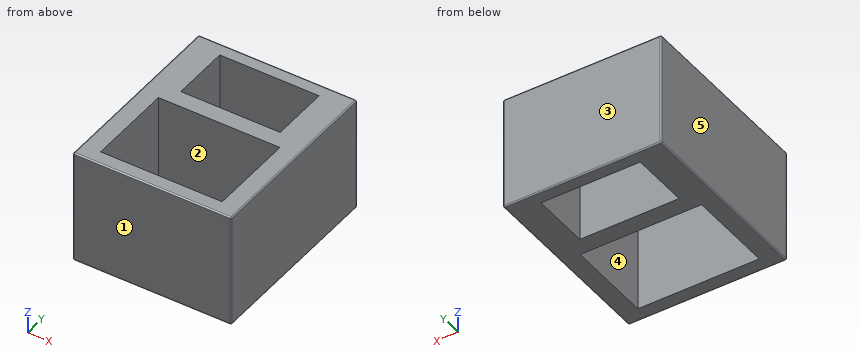
from build123d import *

# Parameters (mm, degrees)
SKETCH_1_W          = 250
SKETCH_1_H          = 300
EXTRUDE_1_DEPTH     = 180
FILLET_1_R          = 2
CUT_EXTRUDE_1_REACH = 432
SKETCH_2_W          = 157
SKETCH_2_H          = 93
SKETCH_2_W_2        = 192
SKETCH_2_H_2        = 138


with BuildPart() as part:
    # 草图1 → 凸台-拉伸1 (new body)
    with BuildSketch(Plane.XY):
        with Locations((125, 150)):
            Rectangle(SKETCH_1_W, SKETCH_1_H)
    extrude(amount=EXTRUDE_1_DEPTH)

    # 圆角1
    fillet_1_edges = [part.edges().sort_by_distance(p)[0] for p in [
        (250, 150, 180),
        (125, 300, 180),
        (0, 150, 180),
        (125, 300, 0),
        (250, 150, 0),
        (125, 0, 0),
        (0, 150, 0),
        (125, 0, 180),
        (0, 300, 90),
        (250, 300, 90),
        (250, 0, 90),
        (0, 0, 90),
    ]]
    fillet(fillet_1_edges, radius=FILLET_1_R)

    # 草图2 → 切除-拉伸1 (cut, up to next)
    with BuildSketch(Plane.XY.offset(180), mode=Mode.PRIVATE) as cut_extrude_1_sk1:
        with Locations((125, 233.5)):
            Rectangle(SKETCH_2_W, SKETCH_2_H)
    cut_extrude_1_tool1 = extrude(cut_extrude_1_sk1.sketch, amount=-CUT_EXTRUDE_1_REACH, mode=Mode.PRIVATE) & part.part
    # 草图2 → 切除-拉伸1 (cut, up to next)
    with BuildSketch(Plane.XY.offset(180), mode=Mode.PRIVATE) as cut_extrude_1_sk2:
        with Locations((125, 91)):
            Rectangle(SKETCH_2_W_2, SKETCH_2_H_2)
    cut_extrude_1_tool2 = extrude(cut_extrude_1_sk2.sketch, amount=-CUT_EXTRUDE_1_REACH, mode=Mode.PRIVATE) & part.part
    add(cut_extrude_1_tool1.solids().sort_by_distance((125, 233.5, 180))[0], mode=Mode.SUBTRACT)
    add(cut_extrude_1_tool2.solids().sort_by_distance((125, 91, 180))[0], mode=Mode.SUBTRACT)


solid = part.part
Model file for the job. Use its own axes, mm. Face numbers are marked on the shaded views. A direction names the side the tool comes from. Round coordinates to 2 decimals unless told otherwise and drop trailing zeros. Order: outer loops, then holes, each group sorted by start corner. A loop starts at its lowest first (then second) coordinate and runs counter-clockwise, first axis right, second up.
(1) Band-saw the part on C-C (z = 114). List the corners of the cut face in (x, y), then the cut area to 3 significant figures.
(2) Band-saw the part on D-D (x = 42.5). List the corners of the cut face in (y, z).
(3) Band-saw the part on A-A (y = 99). List the corners of the cut face in (x, z), then the cut area to 3 significant figures.
(4) 3-axis set-ups, long thin cutter, end or side, ignore diameter. For the marked faces 1 and 2: which of +Z, -Z, +X, -X, +Y, -Y reach the whole face in a straight line?
(5) Pull direction Y, two halves, no side cores. Call the marked faces 3, 4 and 5: released by +Y, released by -Y, zero draft, split by the parting line, or undercut.
(6) Drill centre lines: line 1 (Y direction, x = 68.5, z = 85.5); line 2 (X direction, y = 266, z = 61.5); line 3 (X direction, y = 51.5, z = 95.5). Where is each one in solid material? Low to high.
(7) Band-saw the part on B-B (x = 121). List the corners of the cut face in (y, z).
Verdict:
1. outline: (0, 2) arc R2 ccw to (2, 0) - (248, 0) arc R2 ccw to (250, 2) - (250, 298) arc R2 ccw to (248, 300) - (2, 300) arc R2 ccw to (0, 298) - close; hole (29, 22) - (221, 22) - (221, 160) - (29, 160) - close; hole (46.5, 187) - (203.5, 187) - (203.5, 280) - (46.5, 280) - close
1. area: 33,900 mm2
2. outline: (0, 2) arc R2 ccw to (2, 0) - (22, 0) - (22, 180) - (2, 180) arc R2 ccw to (0, 178) - close; (160, 0) - (298, 0) arc R2 ccw to (300, 2) - (300, 178) arc R2 ccw to (298, 180) - (160, 180) - close
3. outline: (0, 2) arc R2 ccw to (2, 0) - (29, 0) - (29, 180) - (2, 180) arc R2 ccw to (0, 178) - close; (221, 0) - (248, 0) arc R2 ccw to (250, 2) - (250, 178) arc R2 ccw to (248, 180) - (221, 180) - close
3. area: 10,400 mm2
4. face 1: +Z, -Z, +X, -X, -Y
4. face 2: +Z, -Z
5. face 3: released by +Y
5. face 4: undercut
5. face 5: zero draft
6. line 1: y = 0 to 22, 160 to 187, 280 to 300
6. line 2: x = 0 to 46.5, 203.5 to 250
6. line 3: x = 0 to 29, 221 to 250
7. outline: (0, 2) arc R2 ccw to (2, 0) - (22, 0) - (22, 180) - (2, 180) arc R2 ccw to (0, 178) - close; (160, 0) - (187, 0) - (187, 180) - (160, 180) - close; (280, 0) - (298, 0) arc R2 ccw to (300, 2) - (300, 178) arc R2 ccw to (298, 180) - (280, 180) - close
